Autodesk Inventor part; units mm, degrees
ref_plane "YZ Plane" through (0, 0, 0) normal (1, 0, 0) x (0, 1, 0)
ref_plane "XZ Plane" through (0, 0, 0) normal (0, 1, 0) x (-1, 0, 0)
ref_plane "XY Plane" through (0, 0, 0) normal (0, 0, 1) x (1, 0, 0)
sketch "Эскиз1" plane through (0, 0, 0) normal (0, 0, 1) x (1, 0, 0)
  circle A0 centre (0, 0) radius 2.5
  circle A1 centre (0, 0) radius 5
  dimension "d0" = 5
  dimension "d1" = 10
extrude "Выдавливание1" add sketch "Эскиз1" along normal mid plane 4
sketch "Эскиз2" plane through (0, 0, 2) normal (0, 0, 1) x (1, 0, 0)
  circle A0 centre (0, 0) radius 4.65
  circle A1 centre (0, 0) radius 3
  dimension "d4" = 9.3
  dimension "d5" = 6
extrude "Выдавливание2" cut sketch "Эскиз2" against normal blind 0.2
sketch "Эскиз3" plane through (0, 0, -2) normal (0, 0, -1) x (-1, 0, 0)
  circle A0 centre (0, 0) radius 3
  circle A1 centre (0, 0) radius 4.65
  dimension "d8" = 6
  dimension "d9" = 9.3
extrude "Выдавливание3" cut sketch "Эскиз3" against normal blind 0.2
properties part number "mr105zz"
Check sheet for the modelled part. Datum: model origin and axes. Units: mm. A direction names the side the tool comes from. Coordinates: 2 decimals unless noted, no trailing zeros. Order: outer loops, then holes, each group sorted by start corner. A loop starts at its lowest first (then second) coordinate and runs counter-clockwise, first axis right, second up. Notation, with made-up numbers: (50, -12.75) -> (63, -12.75) arc R35 cw to (63, 26.25) -> close; hole circle Ø2 at (6, 88). An arc over 180 degrees is marked (long way). Write item = value, one per line. Start each with the question number.
1) Cross-section at B-B (y = -2). Enter the section's corners in (x, z).
2) Material ranges on L1, parallel to Y at x = 0, z = 1.95; L2, parallel to Y at x = 0, z = 0.2; L3, parallel to Z at x = 1, y = 3.5, recorded low to high.
3) Mould release check, pull along Y, two halves, no side actions. Record for faces 1 (the flat face through (-2, 2, -2)), 2 (the cylindrical face through (-1.08, -4.88, 0.03)), 3 (the cylindrical face through (-0.54, 2.44, -0.03)): +Y half, -Y half, draft (parallel to the pull), parting line (faces both ways), or undercut.
4) Go/stop test with a flat-tipped pin: P1, Ø1.5, axis at y = 3.5, z = -1.5, coming from the -X side. Record where the tip stops, or that it passes through.
5) Cross-section at D-D (z = -1.2). Enter the section's corners in (x, y).
6) Cross-section at A-A (x = 0). Enter the section's corners in (y, z), then the cut area to 3 significant figures.
7) Access from +Z, -Z, +X, -X, +Y, -Y to the whole of each face (thin tool, end or side, straight path). Record for faces 4 (the flat face through (-2, 2, 2)), 5 (the flat face through (3, -1, 1.8)), 6 (the flat face through (-3, -1, -1.8)).
8) Cross-section at C-C (y = 4.25). Enter the section's corners in (x, z).
Ans:
q1.outline = (-4.58, -2) -> (-4.2, -2) -> (-4.2, -1.8) -> (-2.24, -1.8) -> (-2.24, -2) -> (-1.5, -2) -> (-1.5, 2) -> (-2.24, 2) -> (-2.24, 1.8) -> (-4.2, 1.8) -> (-4.2, 2) -> (-4.58, 2) -> close; (1.5, -2) -> (2.24, -2) -> (2.24, -1.8) -> (4.2, -1.8) -> (4.2, -2) -> (4.58, -2) -> (4.58, 2) -> (4.2, 2) -> (4.2, 1.8) -> (2.24, 1.8) -> (2.24, 2) -> (1.5, 2) -> close
q2.L1 = -5 to -4.65, -3 to -2.5, 2.5 to 3, 4.65 to 5
q2.L2 = -5 to -2.5, 2.5 to 5
q2.L3 = -1.8 to 1.8
q3.face_1 = draft
q3.face_2 = parting line
q3.face_3 = undercut
q4.P1 = -4.18
q5.outline = circle Ø10 at (0, 0); hole circle Ø5 at (0, 0)
q6.outline = (-5, -2) -> (-4.65, -2) -> (-4.65, -1.8) -> (-3, -1.8) -> (-3, -2) -> (-2.5, -2) -> (-2.5, 2) -> (-3, 2) -> (-3, 1.8) -> (-4.65, 1.8) -> (-4.65, 2) -> (-5, 2) -> close; (2.5, -2) -> (3, -2) -> (3, -1.8) -> (4.65, -1.8) -> (4.65, -2) -> (5, -2) -> (5, 2) -> (4.65, 2) -> (4.65, 1.8) -> (3, 1.8) -> (3, 2) -> (2.5, 2) -> close
q6.area = 18.7 mm²
q7.face_4 = +Z, +X, -X, +Y, -Y
q7.face_5 = +Z
q7.face_6 = -Z
q8.outline = (-2.63, -2) -> (-1.89, -2) -> (-1.89, -1.8) -> (1.89, -1.8) -> (1.89, -2) -> (2.63, -2) -> (2.63, 2) -> (1.89, 2) -> (1.89, 1.8) -> (-1.89, 1.8) -> (-1.89, 2) -> (-2.63, 2) -> close
